```python
from build123d import *

# Parameters (mm, degrees)
F1_ANGLE = 30
F2_R     = 2
F3_R     = 2
F4_R     = 2.25
F4_R_2   = 3
F5_DEPTH = 424.191445
F6_R     = 3.75
F7_DEPTH = 3
F8_R     = 3.75
F9_DEPTH = 3


with BuildPart() as f1:
    # F0 (on Top) → F1 (revolve)
    with BuildSketch(Plane.XY):
        with BuildLine():
            Line((127, 194.31499), (127, 218.81499))
            ThreePointArc((127, 218.81499), (65.760199, 244.304311), (0, 253))
            Line((0, 253), (0, 246.65))
            ThreePointArc((0, 246.65), (62.544207, 238.588442), (121, 214.930739))
            Line((121, 214.930739), (121, 194.31499))
            Line((121, 194.31499), (127, 194.31499))
        make_face()
        with BuildLine():
            Line((0, 246.65), (0, 253))
            ThreePointArc((0, 253), (-65.760199, 244.304311), (-127, 218.81499))
            Line((-127, 218.81499), (-127, 194.31499))
            Line((-127, 194.31499), (-121, 194.31499))
            Line((-121, 194.31499), (-121, 214.930739))
            ThreePointArc((-121, 214.930739), (-62.544207, 238.588442), (0, 246.65))
        make_face()
    revolve(axis=Axis((69.665767, 0, 0), (1, 0, 0)), revolution_arc=F1_ANGLE)

    # F2
    f2_edges = [f1.edges().sort_by_distance(p)[0] for p in [
        (121, 207.607152, 55.628169),
    ]]
    fillet(f2_edges, radius=F2_R)

    # F3
    f3_edges = [f1.edges().sort_by_distance(p)[0] for p in [
        (-121, 207.607152, 55.628169),
    ]]
    fillet(f3_edges, radius=F3_R)

    # F4 (on face) → F5 (cut, symmetric)
    with BuildSketch(Plane.YZ.offset(-121)):
        with Locations((203.893977, 7.629174)):
            Circle(F4_R)
        with Locations((202.753719, 22.844858)):
            Circle(F4_R_2)
        with Locations((200.47958, 37.932783)):
            Circle(F4_R)
        with Locations((197.084278, 52.808573)):
            Circle(F4_R_2)
        with Locations((192.586801, 67.389036)):
            Circle(F4_R)
        with Locations((187.0123, 81.592633)):
            Circle(F4_R_2)
        with Locations((180.391951, 95.33993)):
            Circle(F4_R)
    extrude(amount=F5_DEPTH, both=True, mode=Mode.SUBTRACT)

    # F6 (on face) → F7 (cut)
    with BuildSketch(Plane.YZ.offset(127)):
        with Locations((203.893977, 7.629174)):
            Circle(F6_R)
        with Locations((200.47958, 37.932783)):
            Circle(F6_R)
        with Locations((192.586801, 67.389036)):
            Circle(F6_R)
        with Locations((180.391951, 95.33993)):
            Circle(F6_R)
    extrude(amount=-F7_DEPTH, mode=Mode.SUBTRACT)

    # F8 (on face) → F9 (cut)
    with BuildSketch(Plane(origin=(-127, 0, 0), x_dir=(0, -1, 0), z_dir=(-1, 0, 0))):
        with Locations((-203.893977, 7.629174)):
            Circle(F8_R)
        with Locations((-200.47958, 37.932783)):
            Circle(F8_R)
        with Locations((-192.586801, 67.389036)):
            Circle(F8_R)
        with Locations((-180.391951, 95.33993)):
            Circle(F8_R)
    extrude(amount=-F9_DEPTH, mode=Mode.SUBTRACT)


solid = f1.part
```
The listing builds one solid part. Answer for the finished solid, in the listing's coordinates (mm). A direction names the side the tool comes from. Round coordinates to 2 decimals unless told otherwise and drop trailing zeros. Use one line per item in the form item = value. Start each with the question number.
1. For a pull along Z with two mould halves and no side action, classify faces 1 (the face through (121, 191, 54)), 2 (the face through (-10, 214.517, 123.852)), 3 (the face through (-124, 199, 36)) as pulls with the +Z half, pulls with the -Z half, needs draft (parallel to the pull), parting line crosses it, or undercut.
2. Given pin 1 Ø12 at (x, z) = (95, 44) entering from +Y; pin 2 Ø6 at (y, z) = (180.39, 95.34) entering from -X; pin 3 Ø3.5 at (y, z) = (202.75, 22.84) entering from +X; pin 4 Ø2 at (y, z) = (194, 69) entering from +X, each flat-ended and moving along its own axis, determine where each tip first touches the part or whether it passes through.
3. A tool of negligible diameter and unlimited length cuts with its end or side. For faces 4 (the face through (125.521, 200.148, 7.794)), 5 (the face through (-125.52, 193.4, 63.73)), 6 (the face through (127, 200, 55)), from which of +Z, -Z, +X, -X, +Y, -Y can it reach the whole face along a straight path? Write none if from no direction.
4. Consider line 1 (X direction, y = 204, z = 53); line 2 (X direction, y = 200.5, z = 115); line 3 (Z direction, x = 54, y = 221). Determine where each line is inside the solid, lowest interval first. Write a range as [from, to].
Geometry check:
q1.face_1 = needs draft
q1.face_2 = pulls with the +Z half
q1.face_3 = undercut
q2.pin_1 = 232.96
q2.pin_2 = -124
q2.pin_3 = through
q2.pin_4 = 124
q3.face_4 = +X
q3.face_5 = -X
q3.face_6 = +Z, -Z, +X, +Y, -Y
q4.line_1 = [-127, -121], [121, 127]
q4.line_2 = [-102.88, -86.09], [86.09, 102.88]
q4.line_3 = [95.28, 110.69]
